from build123d import *

# Parameters (mm, degrees)
BOSS_EXTRUDE1_DEPTH      = 0.7
SKETCH2_W                = 153.84
SKETCH2_H                = 85.63
CUT_EXTRUDE1_DEPTH       = 0.8
SKETCH3_W                = 153.84
SKETCH3_H                = 85.63
BOSS_EXTRUDE4_DEPTH      = 0.75
BOSS_EXTRUDE4_DEPTH_BACK = 0.05
SKETCH4_W                = 164.9
SKETCH4_H                = 100
BOSS_EXTRUDE5_DEPTH      = 4.43
BOSS_EXTRUDE6_DEPTH      = 0.1
BOSS_EXTRUDE7_DEPTH      = 0.2


with BuildPart() as part:
    # Sketch1 → Boss-Extrude1 (new body)
    with BuildSketch(Plane.XY):
        with BuildLine():
            Line((-89.04, 60.96), (89.04, 60.96))
            ThreePointArc((89.04, 60.96), (93.282640687, 59.202640687), (95.04, 54.96))
            Line((95.04, 54.96), (95.04, -54.96))
            ThreePointArc((95.04, -54.96), (93.282640687, -59.202640687), (89.04, -60.96))
            Line((89.04, -60.96), (-89.04, -60.96))
            ThreePointArc((-89.04, -60.96), (-93.282640687, -59.202640687), (-95.04, -54.96))
            Line((-95.04, -54.96), (-95.04, 54.96))
            ThreePointArc((-95.04, 54.96), (-93.282640687, 59.202640687), (-89.04, 60.96))
        make_face()
    extrude(amount=BOSS_EXTRUDE1_DEPTH)

    # Sketch2 → Cut-Extrude1 (cut)
    with BuildSketch(Plane.XY):
        with Locations((0, -0.005)):
            Rectangle(SKETCH2_W, SKETCH2_H)
    extrude(amount=CUT_EXTRUDE1_DEPTH, mode=Mode.SUBTRACT)

    # Sketch3 → Boss-Extrude4 (add, two sides)
    with BuildSketch(Plane.XY) as boss_extrude4_sk:
        with Locations((0, -0.005)):
            Rectangle(SKETCH3_W, SKETCH3_H)
    extrude(amount=BOSS_EXTRUDE4_DEPTH)
    extrude(boss_extrude4_sk.sketch, amount=-BOSS_EXTRUDE4_DEPTH_BACK)

    # Sketch4 → Boss-Extrude5 (add)
    with BuildSketch(Plane.XY.offset(0.7)):
        with Locations((1.49, -2.26)):
            Rectangle(SKETCH4_W, SKETCH4_H)
    extrude(amount=BOSS_EXTRUDE5_DEPTH)

    # Sketch5 → Boss-Extrude6 (add)
    with BuildSketch(Plane.XY.offset(5.13)):
        Polygon((48.995697603, 18.69), (69.995697603, 18.69), (69.995697603, -45.31), (22.995697603, -45.31), (22.995697603, -55.31), (-7.004302397, -55.31), (-7.004302397, -22.31), (48.995697603, -22.31), align=None)
    extrude(amount=BOSS_EXTRUDE6_DEPTH)

    # Sketch6 → Boss-Extrude7 (add)
    with BuildSketch(Plane.XY.offset(5.13)):
        Polygon((32.59, 15.01), (27.09, 15.01), (27.09, -55.31), (46.94, -55.31), (46.94, -10.99), (32.59, -10.99), align=None)
    extrude(amount=BOSS_EXTRUDE7_DEPTH)


solid = part.part
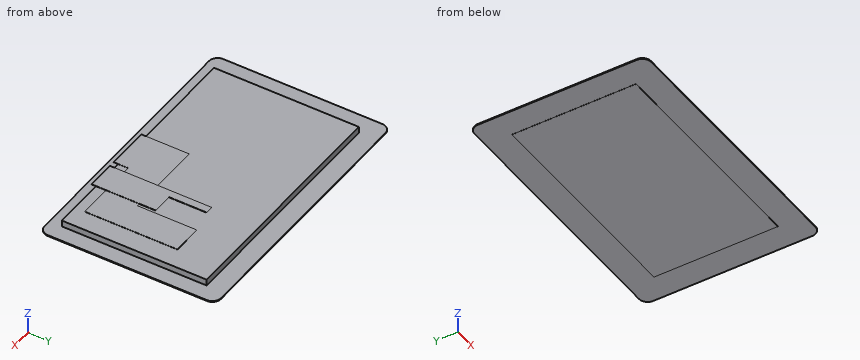
The listing builds one solid part. Answer for the finished solid, in the listing's coordinates (mm). Coordinates: 2 decimals unless noted, no trailing zeros. Order: outer loops, then holes, each group sorted by start corner. A loop starts at its lowest first (then second) coordinate and runs counter-clockwise, first axis right, second up. Notation, with made-up numbers: (18, 38) -> (74, 38) arc R19 cw to (74, 70) -> close; hole circle Ø1 at (34.5, -14.5). An arc over 180 degrees is marked (long way). Answer in a Markdown table with one row per item. Add a question column.
Item 1: Find section A-A (y = 8). Write down the section's boundary in (x, z), then the cut area to 3 significant figures.
Item 2: Find section C-C (z = 3.4). Write down the section's boundary in (x, y).
Item 3: Find section D-D (x = -40). Write down the section's boundary in (y, z).
Item 4: Each of these flat-tipped pins is pushed along its axis until it touches: P1, Ø2, axis at x = 28, z = 4, coming from the -Y side; P2, Ø8, axis at x = -28.5, y = -8, coming from the +Z side; P3, Ø1.3, axis at y = -18.5, z = 3.5, coming from the -X side. Where does it stop, or does it pass through?
Item 5: Find the intervals of material crossed by L1, parallel to X at y = -44.5, z = 2.2; L2, parallel to Y at x = -53, z = 2.85; L3, parallel to Z at x = -85, y = 3.5, in increasing order. Write a range as from..to.
Item 6: Find section B-B (x = 18.5). Write down the section's boundary in (y, z), then the cut area to 3 significant figures.
Result set:
| question | item | result |
|---|---|---|
| 1 | outline | (-95.04, 0) -> (-76.92, 0) -> (-76.92, -0.05) -> (76.92, -0.05) -> (76.92, 0) -> (95.04, 0) -> (95.04, 0.7) -> (83.94, 0.7) -> (83.94, 5.13) -> (70, 5.13) -> (70, 5.23) -> (49, 5.23) -> (49, 5.13) -> (32.59, 5.13) -> (32.59, 5.33) -> (27.09, 5.33) -> (27.09, 5.13) -> (-80.96, 5.13) -> (-80.96, 0.7) -> (-95.04, 0.7) -> close |
| 1 | area | 874 mm² |
| 2 | outline | (-80.96, -52.26) -> (83.94, -52.26) -> (83.94, 47.74) -> (-80.96, 47.74) -> close |
| 3 | outline | (-60.96, 0) -> (-42.82, 0) -> (-42.82, -0.05) -> (42.81, -0.05) -> (42.81, 0) -> (60.96, 0) -> (60.96, 0.7) -> (47.74, 0.7) -> (47.74, 5.13) -> (-52.26, 5.13) -> (-52.26, 0.7) -> (-60.96, 0.7) -> close |
| 4 | P1 | stops at y = -52.26 |
| 4 | P2 | stops at z = 5.13 |
| 4 | P3 | stops at x = -80.96 |
| 5 | L1 | x = -80.96..83.94 |
| 5 | L2 | y = -52.26..47.74 |
| 5 | L3 | z = 0..0.7 |
| 6 | outline | (-60.96, 0) -> (-42.82, 0) -> (-42.82, -0.05) -> (42.81, -0.05) -> (42.81, 0) -> (60.96, 0) -> (60.96, 0.7) -> (47.74, 0.7) -> (47.74, 5.13) -> (-22.31, 5.13) -> (-22.31, 5.23) -> (-55.31, 5.23) -> (-55.31, 5.13) -> (-52.26, 5.13) -> (-52.26, 0.7) -> (-60.96, 0.7) -> close |
| 6 | area | 536 mm² |
